Autodesk Inventor part; units mm, degrees
ref_plane "YZ Plane" through (0, 0, 0) normal (1, 0, 0) x (0, 1, 0)
ref_plane "XZ Plane" through (0, 0, 0) normal (0, 1, 0) x (-1, 0, 0)
ref_plane "XY Plane" through (0, 0, 0) normal (0, 0, 1) x (1, 0, 0)
sketch "Sketch1" plane through (0, 0, 0) normal (0, 1, 0) x (-1, 0, 0)
  line L0 (-10.16, 10.16) -> (10.16, 10.16)
  line L1 (10.16, 10.16) -> (10.16, -10.16)
  line L2 (-10.16, -10.16) -> (-10.16, 10.16)
  circle A0 centre (6.9088, -6.9148) radius 1.9304
  circle A1 centre (6.9088, 6.9088) radius 1.9304
  circle A2 centre (-6.9088, 6.9088) radius 1.9304
  circle A3 centre (-6.9088, -6.9148) radius 1.9304
  line L3 (-5.715, -10.16) -> (-5.715, -20.574)
  line L4 (-5.715, -20.574) -> (6.985, -20.574)
  line L5 (6.985, -20.574) -> (6.985, -10.16)
  line L6 (10.16, -10.16) -> (6.985, -10.16)
  line L7 (-5.715, -10.16) -> (-10.16, -10.16)
  point P0 (0, 0)
  dimension "d0" = 20.32
  dimension "d2" = 10.16
  dimension "d3" = 10.16
  dimension "d4" = 3.8608
  dimension "d5" = 6.9148
  dimension "d6" = 6.9088
  dimension "d7" = 3.8608
  dimension "d8" = 6.9088
  dimension "d9" = 6.9088
  dimension "d10" = 3.8608
  dimension "d11" = 6.9088
  dimension "d12" = 6.9088
  dimension "d13" = 3.8608
  dimension "d14" = 12.7
  dimension "d16" = 6.985
extrude "Extrusion1" add sketch "Sketch1" along normal blind 6.985
sketch "Sketch2" plane through (-6.985, 0, -20.574) normal (-1, 0, 0) x (0, 0, 1)
  circle A0 centre (5.08, 3.4925) radius 4.6609 construction
  line L0 (10.414, 0) -> (0, 0)
  line L1 (0, 0) -> (0, 6.985)
  line L2 (9.7409, 3.4925) -> (7.4105, -0.544)
  line L3 (7.4105, -0.544) -> (2.7496, -0.544)
  line L4 (2.7496, -0.544) -> (0.4191, 3.4925)
  line L5 (0.4191, 3.4925) -> (2.7495, 7.529)
  line L6 (2.7495, 7.529) -> (7.4104, 7.529)
  line L7 (7.4104, 7.529) -> (9.7409, 3.4925)
  point P0 (20.574, 0)
  dimension "d19" = 9.3218
  dimension "d20" = 3.4925
  dimension "d21" = 5.08
extrude "Extrusion2" cut sketch "Sketch2" against normal blind 3.81
sketch "Sketch3" plane through (5.715, 0, -10.16) normal (1, 0, 0) x (0, 0, -1)
  circle A0 centre (5.334, 3.4925) radius 1.9304
  line L0 (10.414, 0) -> (10.414, 6.985)
  line L1 (0, 6.985) -> (10.414, 6.985)
  point P0 (-10.16, 0)
  dimension "d24" = 3.8608
  dimension "d25" = 5.08
  dimension "d26" = 3.4925
extrude "Extrusion3" cut sketch "Sketch3" against normal through all
sketch "Sketch4" plane through (0, 6.985, 0) normal (0, 1, 0) x (1, 0, 0)
  circle A0 centre (0, 0) radius 6.35
  dimension "d29" = 12.7
extrude "Extrusion4" add sketch "Sketch4" along normal blind 2.54
sketch "Sketch5" plane through (0, 9.525, 0) normal (0, 1, 0) x (1, 0, 0)
  arc A0 (1.8926, -2.4892) -> (-1.8926, -2.4892) centre (0, 0) ccw
  line L0 (-1.8926, -2.4892) -> (1.8926, -2.4892)
  dimension "d32" = 6.254
  dimension "d33" = 2.4892
fillet "Fillet1" radius 3.3782 4 edges at (10.16, 3.4925, 10.16) (10.16, 3.4925, -10.16) (-10.16, 3.4925, 10.16) (-10.16, 3.4925, -10.16)
extrude "Extrusion5" cut sketch "Sketch5" against normal through all
sketch "Sketch6" plane through (0, 9.525, 0) normal (0, 1, 0) x (1, 0, 0)
  line L0 (-6.985, 20.574) -> (5.715, 20.574)
  line L1 (0.635, 0) -> (0.635, 20.574)
  line L2 (0.635, 20.574) -> (-0.635, 20.574)
  line L3 (-0.635, 20.574) -> (-0.635, 0)
  line L4 (-0.635, -20.574) -> (0.635, 20.574) construction
  line L5 (0.635, -20.574) -> (-0.635, 20.574) construction
  line L6 (-0.635, 0) -> (0.635, 0)
  point P0 (0, 0)
  dimension "d37" = 1.27
extrude "Extrusion6" cut sketch "Sketch6" against normal through all
properties part number "clamping hub 6mm to 8mm hub"
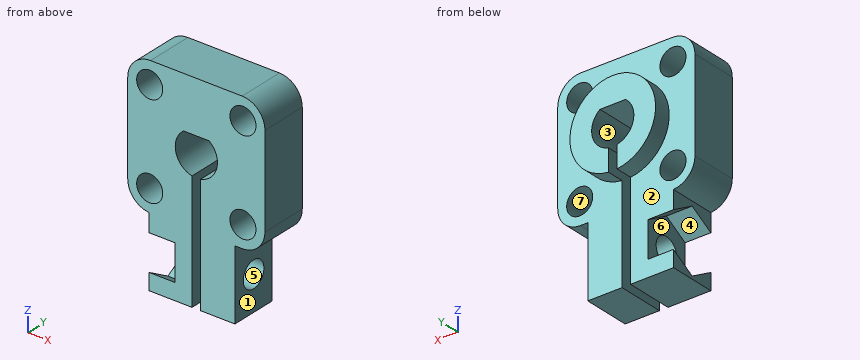
Could you check a few things on this model? Use its own coordinates, in mm. Face numbers are marked on the shaded views. A direction names the side the tool comes from. Give positions to 0.01 mm unless a question says otherwise; leave off trailing zeros. Order: outer loops, then holes, each group sorted by start corner. A loop starts at its lowest first (then second) coordinate and runs counter-clockwise, first axis right, second up.
Q1. If I drill on line 1 along Z through (x, y) = (2.5, 4); line 2 along X through (y, z) = (6, -17.5) (3 decimals); line 3 along X through (y, z) = (5, -4) (3 decimals), over which ranges is the centre line in solid material (lowest first)?
Q2. Suppose I cut it at C-C, the plane x = -7.5. Write out the boundary of the cut face in (y, z) (3 decimals).
Q3. Suppose I cut it at B-B, the plane y = 4. Count the separate pieces of the cut face and the enclosed holes in it, and give its area (3 significant figures).
Q4. I'm going to push flat-ended pins straight in: P1, Ø5.5, axis at y = 3.5, z = -17, coming from the +X side (3 decimals); P2, Ø6, axis at x = 6.91, z = -6.91, coming from the +Y side (3 decimals); P3, Ø1.9, axis at y = 2, z = -19.5, coming from the -X side (3 decimals). Where does each tip first touch, or does it pass through?
Q5. Suppose I cut it at A-A, the plane z = 0. Write out the boundary of the cut face in (x, y) (3 decimals), and give its area (3 significant figures).
Q6. For the marked faces 1, 2, 3 and 4, which set-ups out of +Z, -Z, +X, -X, +Y, -Y let a thin tool reach every point of the face, with its end or its side?
Q7. Suppose I cut it at D-D, the plane z = 6. Write out the boundary of the cut face in (x, y) (3 decimals).
Q8. We'd pull the mould along X, two halves only. Please class the marked faces 5, 6 and 7: +X half, -X half, draft (parallel to the pull), parting line (faces both ways), or undercut.
Solution:
1. line 1: z = -20.57 to -17.36, -13.63 to -1.88, 1.88 to 10.16
1. line 2: x = -3.175 to -0.635, 0.635 to 5.715
1. line 3: x = -10.16 to -0.635, 0.635 to 10.16
2. outline: (0, -10.083) - (6.985, -10.083) - (6.985, -8.752) - (0, -8.752) - close; (0, -5.077) - (6.985, -5.077) - (6.985, 5.071) - (0, 5.071) - close; (0, 8.746) - (6.985, 8.746) - (6.985, 10.083) - (0, 10.083) - close
3. separate pieces: 3
3. enclosed holes: 4
3. area: 376 mm2
4. P1: stops at x = 5.715
4. P2: stops at y = 6.985
4. P3: stops at x = -6.985
5. outline: (-10.16, 0) - (-3.127, 0) - (-3.127, 9.525) - (-6.35, 9.525) - (-6.35, 6.985) - (-10.16, 6.985) - close; (3.127, 0) - (10.16, 0) - (10.16, 6.985) - (6.35, 6.985) - (6.35, 9.525) - (3.127, 9.525) - close
5. area: 115 mm2
6. face 1: -Z, +X, +Y, -Y
6. face 2: +Y
6. face 3: +Y, -Y
6. face 4: -X
7. outline: (-10.16, 0) - (-8.612, 0) - (-8.612, 6.985) - (-10.16, 6.985) - close; (-5.206, 0) - (5.206, 0) - (5.206, 6.985) - (2.079, 6.985) - (2.079, 9.525) - (-2.079, 9.525) - (-2.079, 6.985) - (-5.206, 6.985) - close; (8.612, 0) - (10.16, 0) - (10.16, 6.985) - (8.612, 6.985) - close
8. face 5: draft
8. face 6: -X half
8. face 7: undercut
